Autodesk Inventor part; units mm, degrees
ref_plane "YZ Plane" through (0, 0, 0) normal (1, 0, 0) x (0, 1, 0)
ref_plane "XZ Plane" through (0, 0, 0) normal (0, 1, 0) x (-1, 0, 0)
ref_plane "XY Plane" through (0, 0, 0) normal (0, 0, 1) x (1, 0, 0)
sketch "草图1" plane through (0, 0, 0) normal (0, 1, 0) x (-1, 0, 0)
  line L0 (200, 200) -> (-200, 200)
  line L1 (-200, 200) -> (-200, -200)
  line L2 (-200, -200) -> (200, -200)
  line L3 (200, -200) -> (200, 200)
  point P0 (0, 0)
  dimension "d0" = 400
  dimension "d1" = 400
extrude "拉伸1" add sketch "草图1" along normal blind 5
sketch "草图2" plane through (0, 5, 0) normal (0, 1, 0) x (1, 0, 0)
  circle A0 centre (175, 175) radius 1.8
  point P0 (0, 0)
  dimension "d4" = 3.6
extrude "拉伸2" cut sketch "草图2" against normal through all
sketch "草图3" plane through (0, 5, 0) normal (0, 1, 0) x (1, 0, 0)
  circle A0 centre (175, -175) radius 1.8
  point P0 (0, 0)
  dimension "d7" = 3.6
extrude "拉伸3" cut sketch "草图3" against normal through all
sketch "草图4" plane through (0, 0, 0) normal (0, -1, 0) x (1, 0, 0)
  circle A0 centre (-175, 175) radius 1.8
  point P0 (0, 0)
  dimension "d10" = 3.6
extrude "拉伸4" cut sketch "草图4" against normal through all
sketch "草图5" plane through (0, 0, 0) normal (0, -1, 0) x (1, 0, 0)
  circle A0 centre (-175, -175) radius 1.8
  point P0 (0, 0)
  dimension "d13" = 3.6
extrude "拉伸5" cut sketch "草图5" against normal through all
sketch "草图8" plane through (0, 5, 0) normal (0, 1, 0) x (1, 0, 0)
  circle A0 centre (-21.4, 185) radius 1.8
  point P0 (0, 0)
  dimension "d24" = 3.6
extrude "拉伸8" cut sketch "草图8" against normal through all
sketch "草图9" plane through (0, 5, 0) normal (0, 1, 0) x (1, 0, 0)
  circle A0 centre (21.4, 185) radius 1.8
  point P0 (0, 0)
  dimension "d27" = 3.6
extrude "拉伸9" cut sketch "草图9" against normal through all
sketch "草图10" plane through (0, 5, 0) normal (0, 1, 0) x (1, 0, 0)
  circle A0 centre (-21.4, 173) radius 1.8
  point P0 (0, 0)
  dimension "d30" = 3.6
extrude "拉伸10" cut sketch "草图10" against normal through all
sketch "草图11" plane through (0, 5, 0) normal (0, 1, 0) x (1, 0, 0)
  circle A0 centre (21.4, 173) radius 1.8
  point P0 (0, 0)
  dimension "d33" = 3.6
extrude "拉伸11" cut sketch "草图11" against normal through all
sketch "草图12" plane through (0, 5, 0) normal (0, 1, 0) x (1, 0, 0)
  circle A0 centre (21.4, -173) radius 1.8
  point P0 (0, 0)
  dimension "d36" = 3.6
extrude "拉伸12" cut sketch "草图12" against normal through all
sketch "草图13" plane through (0, 5, 0) normal (0, 1, 0) x (1, 0, 0)
  circle A0 centre (21.4, -185) radius 1.8
  point P0 (0, 0)
  dimension "d39" = 3.6
extrude "拉伸13" cut sketch "草图13" against normal through all
sketch "草图14" plane through (0, 5, 0) normal (0, 1, 0) x (1, 0, 0)
  circle A0 centre (-21.4, -185) radius 1.8
  point P0 (0, 0)
  dimension "d42" = 3.6
extrude "拉伸14" cut sketch "草图14" against normal through all
sketch "草图15" plane through (0, 5, 0) normal (0, 1, 0) x (1, 0, 0)
  circle A0 centre (-21.4, -173) radius 1.8
  point P0 (0, 0)
  dimension "d45" = 3.6
extrude "拉伸15" cut sketch "草图15" against normal through all
sketch "草图16" plane through (0, 5, 0) normal (0, 1, 0) x (1, 0, 0)
  circle A0 centre (50, 160) radius 5
  point P0 (0, 0)
  dimension "d48" = 10
extrude "拉伸16" cut sketch "草图16" against normal through all
sketch "草图17" plane through (0, 0, 0) normal (0, -1, 0) x (1, 0, 0)
  circle A0 centre (-50, 160) radius 5
  point P0 (0, 0)
  dimension "d51" = 10
extrude "拉伸17" cut sketch "草图17" against normal through all
sketch "草图18" plane through (0, 0, 0) normal (0, -1, 0) x (1, 0, 0)
  circle A0 centre (-50, -160) radius 5
  point P0 (0, 0)
  dimension "d54" = 10
extrude "拉伸18" cut sketch "草图18" against normal through all
sketch "草图19" plane through (0, 0, 0) normal (0, -1, 0) x (1, 0, 0)
  circle A0 centre (50, 160) radius 5
  point P0 (0, 0)
  dimension "d57" = 10
extrude "拉伸19" cut sketch "草图19" against normal through all
sketch "草图20" plane through (0, 5, 0) normal (0, 1, 0) x (1, 0, 0)
  point P0 (0, 0)
sketch "草图21" plane through (0, 5, 0) normal (0, 1, 0) x (1, 0, 0)
  point P0 (0, 0)
sketch "草图22" plane through (0, 5, 0) normal (0, 1, 0) x (1, 0, 0)
  circle A0 centre (195, -85) radius 1.8
  point P0 (0, 0)
  dimension "d60" = 3.6
extrude "拉伸20" cut sketch "草图22" against normal through all
sketch "草图23" plane through (0, 5, 0) normal (0, 1, 0) x (1, 0, 0)
  circle A0 centre (171, -85) radius 1.8
  point P0 (0, 0)
  dimension "d63" = 3.6
extrude "拉伸21" cut sketch "草图23" against normal through all
sketch "草图27" plane through (0, 5, 0) normal (0, 1, 0) x (1, 0, 0)
  circle A0 centre (-195, 85) radius 1.8
  point P0 (0, 0)
  dimension "d75" = 3.6
extrude "拉伸25" cut sketch "草图27" against normal through all
sketch "草图28" plane through (0, 5, 0) normal (0, 1, 0) x (1, 0, 0)
  circle A0 centre (-171, 85) radius 1.8
  point P0 (0, 0)
  dimension "d78" = 3.6
extrude "拉伸26" cut sketch "草图28" against normal through all
sketch "草图30" plane through (0, 0, 0) normal (0, -1, 0) x (1, 0, 0)
  circle A0 centre (171, 55) radius 1.8
  point P0 (0, 0)
  dimension "d85" = 3.6
extrude "拉伸27" cut sketch "草图30" against normal through all
sketch "草图31" plane through (0, 0, 0) normal (0, -1, 0) x (1, 0, 0)
  circle A0 centre (195, 55) radius 1.8
  point P0 (0, 0)
  dimension "d88" = 3.6
extrude "拉伸28" cut sketch "草图31" against normal through all
sketch "草图32" plane through (0, 0, 0) normal (0, -1, 0) x (1, 0, 0)
  circle A0 centre (-195, -55) radius 1.8
  point P0 (0, 0)
  dimension "d91" = 3.6
extrude "拉伸29" cut sketch "草图32" against normal through all
sketch "草图33" plane through (0, 0, 0) normal (0, -1, 0) x (1, 0, 0)
  circle A0 centre (-171, 55) radius 1.8
  point P0 (0, 0)
  dimension "d94" = 3.6
extrude "拉伸30" cut sketch "草图33" against normal through all
sketch "草图34" plane through (0, 0, 0) normal (0, -1, 0) x (1, 0, 0)
  circle A0 centre (-171, -55) radius 1.8
  point P0 (0, 0)
  dimension "d97" = 3.6
extrude "拉伸31" cut sketch "草图34" against normal through all
sketch "草图35" plane through (0, 0, 0) normal (0, -1, 0) x (1, 0, 0)
  circle A0 centre (-195, 55) radius 1.8
  point P0 (0, 0)
  dimension "d100" = 3.6
extrude "拉伸32" cut sketch "草图35" against normal through all
sketch "草图36" plane through (0, 0, 0) normal (0, -1, 0) x (1, 0, 0)
  circle A0 centre (-171, 85) radius 1.8
  point P0 (0, 0)
  dimension "d103" = 3.6
extrude "拉伸33" cut sketch "草图36" against normal through all
sketch "草图37" plane through (0, 0, 0) normal (0, -1, 0) x (1, 0, 0)
  circle A0 centre (-195, 85) radius 1.8
  point P0 (0, 0)
  dimension "d106" = 3.6
extrude "拉伸34" cut sketch "草图37" against normal through all
sketch "草图38" plane through (0, 0, 0) normal (0, -1, 0) x (1, 0, 0)
  circle A0 centre (195, -55) radius 1.8
  point P0 (0, 0)
  dimension "d109" = 3.6
extrude "拉伸35" cut sketch "草图38" against normal through all
sketch "草图39" plane through (0, 0, 0) normal (0, -1, 0) x (1, 0, 0)
  circle A0 centre (171, -55) radius 1.8
  point P0 (0, 0)
  dimension "d112" = 3.6
extrude "拉伸36" cut sketch "草图39" against normal through all
sketch "草图40" plane through (0, 0, 0) normal (0, -1, 0) x (1, 0, 0)
  circle A0 centre (171, -85) radius 1.8
  point P0 (0, 0)
  dimension "d115" = 3.6
extrude "拉伸37" cut sketch "草图40" against normal through all
sketch "草图41" plane through (0, 0, 0) normal (0, -1, 0) x (1, 0, 0)
  circle A0 centre (195, -85) radius 1.8
  point P0 (0, 0)
  dimension "d118" = 3.6
extrude "拉伸38" cut sketch "草图41" against normal through all
sketch "草图42" plane through (0, 0, 0) normal (0, -1, 0) x (1, 0, 0)
  circle A0 centre (65, 156) radius 1.8
  point P0 (0, 0)
  dimension "d121" = 3.6
extrude "拉伸39" cut sketch "草图42" against normal through all
sketch "草图43" plane through (0, 0, 0) normal (0, -1, 0) x (1, 0, 0)
  circle A0 centre (95, 156) radius 1.8
  point P0 (0, 0)
  dimension "d124" = 3.6
extrude "拉伸40" cut sketch "草图43" against normal through all
sketch "草图44" plane through (0, 0, 0) normal (0, -1, 0) x (1, 0, 0)
  circle A0 centre (65, 180) radius 1.8
  point P0 (0, 0)
  dimension "d127" = 3.6
extrude "拉伸41" cut sketch "草图44" against normal through all
sketch "草图45" plane through (0, 5, 0) normal (0, 1, 0) x (1, 0, 0)
  circle A0 centre (95, -180) radius 1.8
  point P0 (0, 0)
  dimension "d130" = 3.6
extrude "拉伸42" cut sketch "草图45" against normal through all
sketch "草图46" plane through (0, 0, 0) normal (0, -1, 0) x (1, 0, 0)
  circle A0 centre (65, -156) radius 1.8
  point P0 (0, 0)
  dimension "d133" = 3.6
extrude "拉伸43" cut sketch "草图46" against normal through all
sketch "草图47" plane through (0, 0, 0) normal (0, -1, 0) x (1, 0, 0)
  circle A0 centre (95, -156) radius 1.8
  point P0 (0, 0)
  dimension "d136" = 3.6
extrude "拉伸44" cut sketch "草图47" against normal through all
sketch "草图48" plane through (0, 0, 0) normal (0, -1, 0) x (1, 0, 0)
  circle A0 centre (65, -180) radius 1.8
  point P0 (0, 0)
  dimension "d139" = 3.6
extrude "拉伸45" cut sketch "草图48" against normal through all
sketch "草图49" plane through (0, 0, 0) normal (0, -1, 0) x (1, 0, 0)
  circle A0 centre (95, -180) radius 1.8
  point P0 (0, 0)
  dimension "d142" = 3.6
extrude "拉伸46" cut sketch "草图49" against normal through all
sketch "草图50" plane through (0, 0, 0) normal (0, -1, 0) x (1, 0, 0)
  circle A0 centre (-95, 156) radius 1.8
  point P0 (0, 0)
  dimension "d145" = 3.6
extrude "拉伸47" cut sketch "草图50" against normal through all
sketch "草图51" plane through (0, 0, 0) normal (0, -1, 0) x (1, 0, 0)
  circle A0 centre (-65, 156) radius 1.8
  point P0 (0, 0)
  dimension "d148" = 3.6
extrude "拉伸48" cut sketch "草图51" against normal through all
sketch "草图52" plane through (0, 0, 0) normal (0, -1, 0) x (1, 0, 0)
  circle A0 centre (-95, 180) radius 1.8
  point P0 (0, 0)
  dimension "d151" = 3.6
extrude "拉伸49" cut sketch "草图52" against normal through all
sketch "草图53" plane through (0, 0, 0) normal (0, -1, 0) x (1, 0, 0)
  circle A0 centre (-65, 180) radius 1.8
  point P0 (0, 0)
  dimension "d154" = 3.6
extrude "拉伸50" cut sketch "草图53" against normal through all
sketch "草图54" plane through (0, 0, 0) normal (0, -1, 0) x (1, 0, 0)
  circle A0 centre (-65, -156) radius 1.8
  point P0 (0, 0)
  dimension "d157" = 3.6
extrude "拉伸51" cut sketch "草图54" against normal through all
sketch "草图55" plane through (0, 0, 0) normal (0, -1, 0) x (1, 0, 0)
  circle A0 centre (-65, -180) radius 1.8
  point P0 (0, 0)
  dimension "d160" = 3.6
extrude "拉伸52" cut sketch "草图55" against normal through all
sketch "草图56" plane through (0, 0, 0) normal (0, -1, 0) x (1, 0, 0)
  circle A0 centre (-95, -156) radius 1.8
  point P0 (0, 0)
  dimension "d163" = 3.6
extrude "拉伸53" cut sketch "草图56" against normal through all
sketch "草图57" plane through (0, 0, 0) normal (0, -1, 0) x (1, 0, 0)
  circle A0 centre (-95, -180) radius 1.8
  point P0 (0, 0)
  dimension "d166" = 3.6
extrude "拉伸54" cut sketch "草图57" against normal through all
sketch "草图58" plane through (0, 0, 0) normal (0, -1, 0) x (1, 0, 0)
  point P0 (0, 0)
properties part number "上层板"
Geometry: final body of the model. Coordinates: model frame, mm. Give positions to 0.01 mm unless a question says otherwise; leave off trailing zeros. Answer as CSV lines item,"result". Start each with the question number.
1. Ray query, L1, parallel to X at y = 2.15, z = 85; L2, parallel to X at y = 3.3, z = -175; L3, parallel to Z at x = -65, y = 1.5. Return the intervals inside material, ascending.
2. Draft query along X for faces 1 (the face through (3, 0, 3)), 2 (the face through (45, 2, 160)). Return one class per face: released by +X, released by -X, zero draft, split by the parting line, or undercut.
3. Pin query (flat end, axial travel): P1, Ø16, axis at x = -50, z = -160, coming from the -Y side. Return the tip coordinate at first contact, or that it passes through.
Answers:
1,L1,"x = -200 to -196.8, -193.2 to -172.8, -169.2 to 169.2, 172.8 to 193.2, 196.8 to 200"
1,L2,"x = -200 to -176.8, -173.2 to 173.2, 176.8 to 200"
1,L3,"z = -200 to -181.8, -178.2 to -157.8, -154.2 to 154.2, 157.8 to 178.2, 181.8 to 200"
2,face 1,"zero draft"
2,face 2,"undercut"
3,P1,"stops at y = 0"
